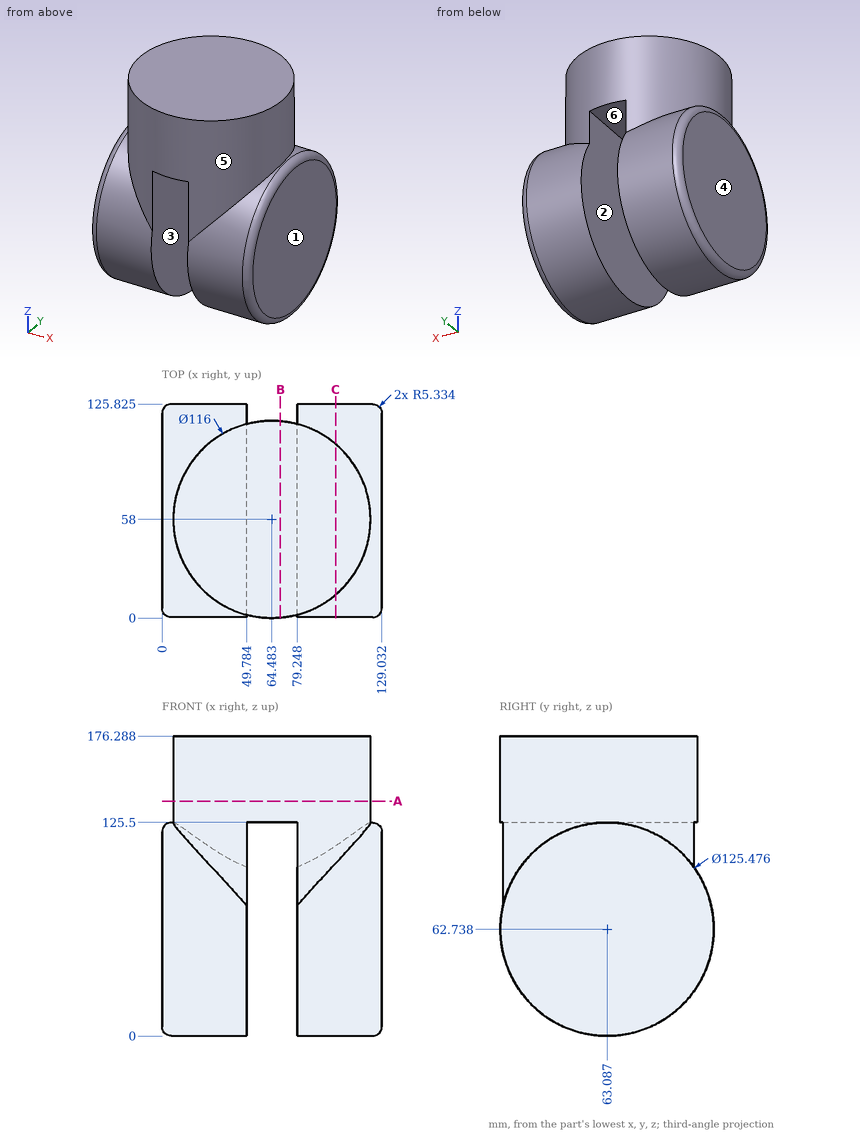
Drawing for the job (mm, zero at the part's lowest x, y, z). A direction names the side the tool comes from. Round coordinates to 2 decimals unless told otherwise and drop trailing zeros. Write each loop counter-clockwise with the first axis right and the second up, starting at its lowest first coordinate (ties: lowest second). Pieces come first, ordered by that corner, then holes. Notation, with made-up numbers: M 51,7 L 60,7 A24 cw 60,42 Z; hole C 19.25,19 d7. An arc over 180 degrees is marked long. Answer as a JSON object with one key per item and string values. Group by question number.
(1) Cut at B-B (x = 69.5). Give the cut face in (y, z).
(2) Flat gauge pins, fed straight in: pin 1 (8 mm diameter, centred on x = 42.5, z = 95.5, fed in from -Y); pin 2 (6 mm diameter, centred on x = 77.5, z = 43.5, fed in from +Y); pin 3 (14.5 mm diameter, centred on x = 64, y = 62.5, fed in from -Z); pin 4 (2 mm diameter, centred on x = 107.5, y = 19, fed in from +Z). Where does each tip first touch, or does it go through?
(3) Cut at C-C (x = 102). Give the cut face in (y, z) (3 decimals), and give its area (3 significant figures).
(4) Which spindle directions (+Z, -Z, +X, -X, +Y, -Y) get a long thin tool onto all of the face, cutting with end or side? Do the marked faces 1 and 2. Say none if no direction does.
(5) Mould opens along X. For the marked faces 3, 4, 5 and 6 say: pulls with the +X half, pulls with the -X half, needs draft (parallel to the pull), parting line crosses it, or undercut.
(6) Drill centre lines: L1, parallel to X at y = 45, z = 27.5; L2, parallel to Z at x = 74, y = 47; L3, parallel to X at y = 59.5, z = 152. Where is each one in solid material? Low to high.
(7) Cut at A-A (z = 138). Give the cut face in (x, y), and give its area (3 significant figures).
Responses:
{
 "1": {"outline": "M 0.22,125.5 L 115.78,125.5 L 115.78,176.29 L 0.22,176.29 Z"},
 "2": {"pin 1": "stops at y = 2.86", "pin 2": "stops at y = 123.53", "pin 3": "stops at z = 125.5", "pin 4": "stops at z = 176.29"},
 "3": {"outline": "M 13.768,101.515 A62.738 ccw long 102.232,111.766 L 102.232,176.288 L 13.768,176.288 Z", "area": "17,400 mm2"},
 "4": {"face 1": "+Z, -Z, +X, +Y, -Y", "face 2": "-Z, +Y, -Y"},
 "5": {"face 3": "undercut", "face 4": "pulls with the -X half", "face 5": "parting line crosses it", "face 6": "undercut"},
 "6": {"L1": "x = 0 to 49.78, 79.25 to 129.03", "L2": "z = 125.5 to 176.29", "L3": "x = 6.5 to 122.46"},
 "7": {"outline": "C 64.48,58 d116", "area": "10,600 mm2"}
}
